The listing builds one solid part. Answer for the finished solid, in the listing's coordinates (mm). Face numbers are marked on the shaded views. A direction names the side the tool comes from. Give positions to 0.01 mm unless a question says otherwise; leave off trailing zeros. Loops run counter-clockwise (first coordinate to the right, second up) from the corner with the lowest first, then second, coordinate; pieces in that order, holes last.
Item 1: Section A-A, the plane x = 0 is taken. Give the vertices of the cut face in (y, z).
Item 2: Consider line 1 along Z through (x, y) = (5.5, -8); line 2 along Y through (x, z) = (0.5, -5); line 3 along Y through (x, z) = (0, -8). Determine where each line is inside the solid, lowest interval first.
Item 3: Section D-D, the plane z = 3.5 is taken. Give the vertices of the cut face in (x, y), and give its area (3 significant figures).
Item 4: A tool of negligible diameter and unlimited length cuts with its end or side. For the marked faces 1 and 2, from which of +Z, -Z, +X, -X, +Y, -Y can it reach the whole face along a straight path? Write none if from no direction.
Item 5: Section C-C, the plane z = 16 is taken. Give the vertices of the cut face in (x, y), and give its area (3 significant figures).
Item 6: Each of these flat-tipped pins is pushed along its axis until it touches: pin 1 Ø12 at (y, z) = (-9.5, 11.5) entering from +X; pin 2 Ø3 at (x, y) = (5.2, -3) entering from +Z; pin 3 Ø4 at (x, z) = (-7.5, -0.5) entering from -Y. Where does it stop, or does it pass through?
Item 7: Section B-B, the plane y = 0 is taken. Give the vertices of the cut face in (x, z), and give its area (4 significant figures).
from build123d import *

# Parameters (mm, degrees)
BOSS_EXTRUDE1_DEPTH      = 15
BOSS_EXTRUDE1_DEPTH_BACK = 10
SKETCH1_R                = 15
FILLET1_R                = 5
SKETCH2_R                = 2.5
BOSS_EXTRUDE2_DEPTH      = 10
CHAMFER1_SIZE            = 0.2
SKETCH3_R                = 1
CUT_EXTRUDE1_DEPTH       = 3
CIRPATTERN1_COUNT        = 3


with BuildPart() as part:
    # Sketch1 → Boss-Extrude1 (new, two sides: drawn at the far end of the back side and taken through both)
    with BuildSketch(Plane.XY.offset(-BOSS_EXTRUDE1_DEPTH_BACK)):
        Circle(SKETCH1_R)
    extrude(amount=BOSS_EXTRUDE1_DEPTH + BOSS_EXTRUDE1_DEPTH_BACK)

    # Fillet1
    fillet1_edges = [part.edges().sort_by_distance(p)[0] for p in [
        (-15, 0, -10),
        (-15, 0, 15),
    ]]
    fillet(fillet1_edges, radius=FILLET1_R)

    # Sketch2 → Boss-Extrude2 (add)
    with BuildSketch(Plane.XY.offset(15)):
        Circle(SKETCH2_R)
    extrude(amount=BOSS_EXTRUDE2_DEPTH)

    # Chamfer1
    chamfer1_edges = [part.edges().sort_by_distance(p)[0] for p in [
        (-2.5, 0, 25),
    ]]
    chamfer(chamfer1_edges, length=CHAMFER1_SIZE)

    # Sketch3 → Cut-Extrude1 (cut)
    with BuildSketch(Plane(origin=(0, 0, -10), x_dir=(-1, 0, 0), z_dir=(0, 0, -1))):
        with Locations((0, 6)):
            Circle(SKETCH3_R)
    cut_extrude1 = extrude(amount=-CUT_EXTRUDE1_DEPTH, mode=Mode.SUBTRACT)

    # CirPattern1: Cut-Extrude1 ×3 about axis
    cirpattern1_axis = Axis((0, 0, 0), (0, 0, 1))
    for i in range(1, CIRPATTERN1_COUNT):
        add(cut_extrude1.rotate(cirpattern1_axis, i * 360 / CIRPATTERN1_COUNT), mode=Mode.SUBTRACT)


solid = part.part
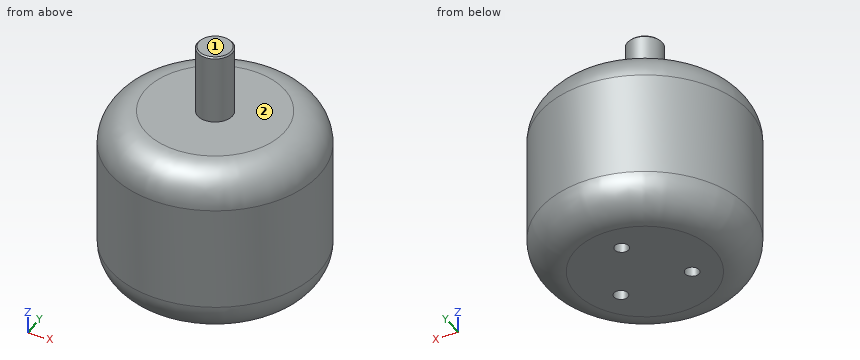
Worked answers:
1. outline: (-15, -5) arc R5 ccw to (-10, -10) - (5, -10) - (5, -7) - (7, -7) - (7, -10) - (10, -10) arc R5 ccw to (15, -5) - (15, 10) arc R5 ccw to (10, 15) - (2.5, 15) - (2.5, 24.8) - (2.3, 25) - (-2.3, 25) - (-2.5, 24.8) - (-2.5, 15) - (-10, 15) arc R5 ccw to (-15, 10) - close
2. line 1: z = -10 to 15
2. line 2: y = -14.99 to 14.99
2. line 3: y = -14 to 5, 7 to 14
3. outline: circle Ø30 at (0, 0)
3. area: 707 mm2
4. face 1: +Z, +X, -X, +Y, -Y
4. face 2: +Z
5. outline: circle Ø5 at (0, 0)
5. area: 19.6 mm2
6. pin 1: stops at x = 14.55
6. pin 2: stops at z = 15
6. pin 3: stops at y = -13.96
7. outline: (-15, -5) arc R5 ccw to (-10, -10) - (10, -10) arc R5 ccw to (15, -5) - (15, 10) arc R5 ccw to (10, 15) - (2.5, 15) - (2.5, 24.8) - (2.3, 25) - (-2.3, 25) - (-2.5, 24.8) - (-2.5, 15) - (-10, 15) arc R5 ccw to (-15, 10) - close
7. area: 778.5 mm2
